```python
from build123d import *

# Parameters (mm, degrees)
SKETCH1_W           = 60
SKETCH1_H           = 30
BOSS_EXTRUDE1_DEPTH = 36.57
CUT_EXTRUDE1_DEPTH  = 60
CUT_EXTRUDE2_REACH  = 82.464
CUT_EXTRUDE3_DEPTH  = 73.14
SKETCH5_R           = 3.75
CUT_EXTRUDE4_DEPTH  = 30
SKETCH6_R           = 7.5
CUT_EXTRUDE5_DEPTH  = 20


with BuildPart() as part:
    # Sketch1 → Boss-Extrude1 (new, symmetric)
    with BuildSketch(Plane.XY):
        Rectangle(SKETCH1_W, SKETCH1_H)
    extrude(amount=BOSS_EXTRUDE1_DEPTH, both=True)

    # Sketch2 → Cut-Extrude1 (cut)
    with BuildSketch(Plane(origin=(30, 0, 0), x_dir=(0, 0, -1), z_dir=(1, 0, 0))):
        with BuildLine():
            ThreePointArc((6, -15), (0, -9), (-6, -15))
            Line((-6, -15), (6, -15))
        make_face()
    extrude(amount=-CUT_EXTRUDE1_DEPTH, mode=Mode.SUBTRACT)

    # Cut-Extrude2: up to this face of the body (flat: up to its plane)
    cut_extrude2_end = Plane(part.part.faces().sort_by_distance((0, 0, -36.57))[0])
    # Sketch3 → Cut-Extrude2 (cut, up to the picked face)
    with BuildSketch(Plane.XY.offset(36.57), mode=Mode.PRIVATE) as cut_extrude2_sk1:
        with BuildLine():
            Line((6.075, 0), (11.075, 0))
            Line((11.075, 0), (15.094237886, -15))
            Line((15.094237886, -15), (-15.094237886, -15))
            Line((-15.094237886, -15), (-11.075, 0))
            Line((-11.075, 0), (-6.075, 0))
            ThreePointArc((-6.075, 0), (0, 6.075), (6.075, 0))
        make_face()
    cut_extrude2_tool1 = split(extrude(cut_extrude2_sk1.sketch, amount=-CUT_EXTRUDE2_REACH, mode=Mode.PRIVATE), bisect_by=cut_extrude2_end, keep=Keep.BOTH, mode=Mode.PRIVATE)
    add(cut_extrude2_tool1.solids().sort_by(Axis((0, -6.537689, 36.57), (0, 0, -1)))[0], mode=Mode.SUBTRACT)

    # Sketch4 → Cut-Extrude3 (cut)
    with BuildSketch(Plane.XY.offset(36.57)):
        Polygon((30, 15), (30, -5), (10, 15), align=None)
        Polygon((-30, 15), (-30, -5), (-10, 15), align=None)
    extrude(amount=-CUT_EXTRUDE3_DEPTH, mode=Mode.SUBTRACT)

    # Sketch5 → Cut-Extrude4 (cut)
    with BuildSketch(Plane(origin=(0, 15, 0), x_dir=(1, 0, 0), z_dir=(0, 1, 0))):
        with Locations(Location((22, -26.57, 0), (0, 0, 180))):
            Circle(SKETCH5_R)
        with Locations(Location((-22, -26.57, 0), (0, 0, 180))):
            Circle(SKETCH5_R)
        with Locations(Location((22, 26.57, 0), (0, 0, 180))):
            Circle(SKETCH5_R)
        with Locations(Location((-22, 26.57, 0), (0, 0, 180))):
            Circle(SKETCH5_R)
    extrude(amount=-CUT_EXTRUDE4_DEPTH, mode=Mode.SUBTRACT)

    # Sketch6 → Cut-Extrude5 (cut)
    with BuildSketch(Plane(origin=(0, 15, 0), x_dir=(1, 0, 0), z_dir=(0, 1, 0))):
        with Locations(Location((22, -26.57, 0), (0, 0, 180))):
            Circle(SKETCH6_R)
        with Locations((-22, -26.57)):
            Circle(SKETCH6_R)
        with Locations(Location((22, 26.57, 0), (0, 0, 180))):
            Circle(SKETCH6_R)
        with Locations(Location((-22, 26.57, 0), (0, 0, 180))):
            Circle(SKETCH6_R)
    extrude(amount=-CUT_EXTRUDE5_DEPTH, mode=Mode.SUBTRACT)


solid = part.part
```
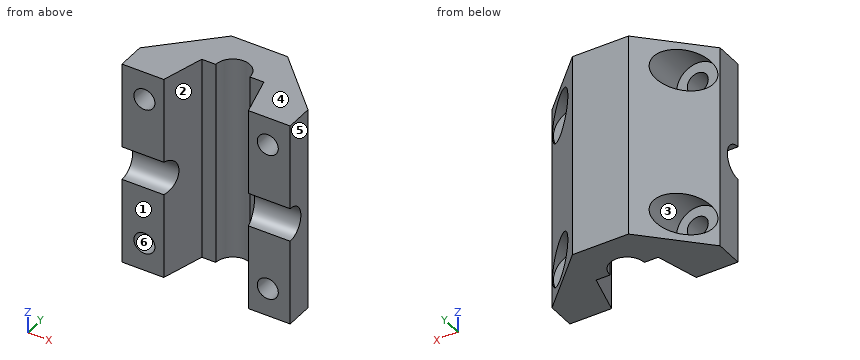
Work out the finished part from the listing and answer in its coordinate system (mm). Face numbers are marked on the shaded views. A direction names the side the tool comes from. Round coordinates to 2 decimals unless told otherwise and drop trailing zeros. Loops run counter-clockwise (first coordinate to the right, second up) from the corner with the lowest first, then second, coordinate; pieces in that order, holes last. Notation, with made-up numbers: (73, -20) -> (111, -20) arc R14 ccw to (111, -1) -> close; hole circle Ø5 at (32.5, -7). An arc over 180 degrees is marked (long way). Write each question's results on one line, items separated by ' | '. Start each with the question number.
1. A tool of negligible diameter and unlimited length cuts with its end or side. For the marked faces 1, 2 and 3, from which of +Z, -Z, +X, -X, +Y, -Y can it reach the whole face along a straight path? Write none if from no direction.
2. Section A-A (z = -26.57) is taken. Determine the outline of the cut face in (x, y) (3 decimals).
3. Section D-D (x = 0) is taken. Determine the outline of the cut face in (y, z) (3 decimals).
4. Section C-C (z = 15.5) is taken. Determine the outline of the cut face in (x, y) (3 decimals).
5. Find the intervals of material crossed by probe 1 along Z at (x, y) = (22, -8); probe 2 along X at (y, z) = (-7, -26); probe 3 along X at (y, z) = (-8, -14), in increasing order. Write a range as from..to.
6. Given pin 1 Ø6 at (x, z) = (-22, 26.57) entering from -Y; pin 2 Ø8.5 at (x, z) = (22, -26.57) entering from -Y; pin 3 Ø7.5 at (x, z) = (23, -25.5) entering from +Y; pin 4 Ø5 at (x, z) = (15, 3) entering from +Y, each flat-ended and moving along its own axis, determine where each tip first touches the part or whether it passes through.
7. For a pull along Z with two mould halves and no side action, classify the marked faces 4, 5 and 6 as +Z half, -Z half, draft (parallel to the pull), parting line (faces both ways), or undercut.
8. Section B-B (x = -22) is taken. Determine the outline of the cut face in (y, z), plus the area to 3 significant figures.
Evaluation:
1) face 1: +Z, -Z, +X, -X, -Y | face 2: +Z, -Z, -Y | face 3: +Y
2) outline: (-30, -15) -> (-25.75, -15) -> (-25.75, -5) -> (-29.5, -5) -> (-29.5, -4.5) -> (-30, -5) -> close; (-18.25, -15) -> (-15.094, -15) -> (-11.075, 0) -> (-6.075, 0) arc R6.075 cw to (6.075, 0) -> (11.075, 0) -> (15.094, -15) -> (18.25, -15) -> (18.25, -5) -> (14.5, -5) -> (14.5, 10.5) -> (10, 15) -> (-10, 15) -> (-14.5, 10.5) -> (-14.5, -5) -> (-18.25, -5) -> close; (25.75, -15) -> (30, -15) -> (30, -5) -> (29.5, -4.5) -> (29.5, -5) -> (25.75, -5) -> close
3) outline: (6.075, -36.57) -> (15, -36.57) -> (15, 36.57) -> (6.075, 36.57) -> close
4) outline: (-30, -15) -> (-15.094, -15) -> (-11.075, 0) -> (-6.075, 0) arc R6.075 cw to (6.075, 0) -> (11.075, 0) -> (15.094, -15) -> (30, -15) -> (30, -5) -> (10, 15) -> (-10, 15) -> (-30, -5) -> close
5) probe 1: z = -36.57..-30.32, -22.82..22.82, 30.32..36.57 | probe 2: x = -30..-25.71, -18.29..-12.95, 12.95..18.29, 25.71..30 | probe 3: x = -30..-13.22, 13.22..30
6) pin 1: passes through | pin 2: stops at y = -15 | pin 3: stops at y = -5 | pin 4: stops at y = 12.5
7) face 4: +Z half | face 5: draft | face 6: undercut
8) outline: (-15, -36.57) -> (3, -36.57) -> (3, -34.07) -> (-5, -34.07) -> (-5, -30.32) -> (-15, -30.32) -> close; (-15, -22.82) -> (-5, -22.82) -> (-5, -19.07) -> (3, -19.07) -> (3, 19.07) -> (-5, 19.07) -> (-5, 22.82) -> (-15, 22.82) -> (-15, 6) arc R6 cw to (-15, -6) -> close; (-15, 30.32) -> (-5, 30.32) -> (-5, 34.07) -> (3, 34.07) -> (3, 36.57) -> (-15, 36.57) -> close | area: 870 mm2
